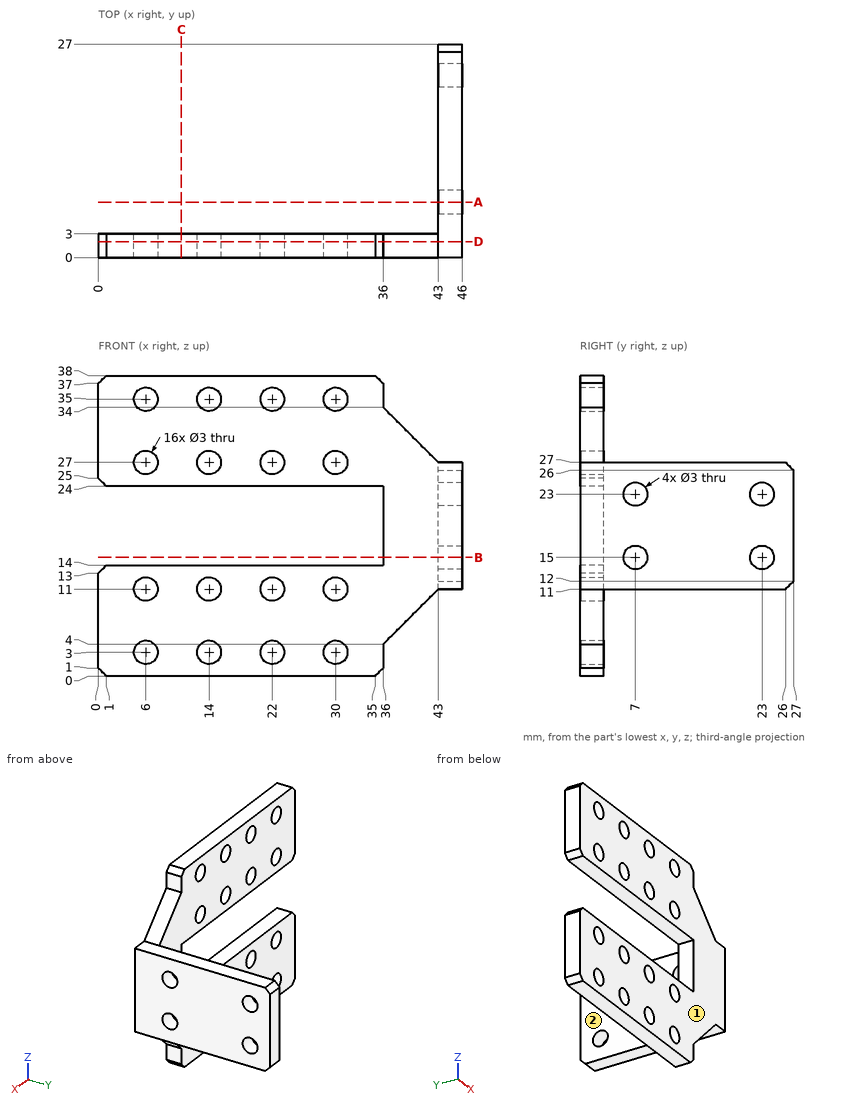
Could you check a few things on this drawing? It's one solid part, dimensions in mm from its lowest x, y, z. A direction names the side the tool comes from. Coordinates: 2 decimals unless noted, no trailing zeros. Loops run counter-clockwise (first coordinate to the right, second up) from the corner with the lowest first, then second, coordinate; pieces in that order, holes last. Notation, with made-up numbers: (77.5, -37) - (104.5, -37) arc R12 cw to (104.5, -30) - close; hole circle Ø11 at (44.25, -16.75). An arc over 180 degrees is marked (long way). Answer as a JSON object with one key per item and string values. Group by question number.
Item 1: If we section it at C-C (x = 10.5): List the corners of the cut face in (y, z) for me.
Item 2: If we section it at A-A (y = 7): List the corners of the cut face in (x, z) for me, plus the area to 3 significant figures.
Item 3: If we section it at D-D (y = 2): State how many separate pieces and enclosed holes the cut face has, plus the area to 3 significant figures.
Item 4: For pin 1 (2.5 mm diameter, centred on x = 30, z = 3, fed in from +Y); pin 2 (0.9 mm diameter, centred on y = 2, z = 16.5, fed in from -X); pin 3 (4 mm diameter, centred on x = 14, z = 11, fed in from +Y); pin 4 (4 mm diameter, centred on x = 22, z = 3, fed in from -Y), each with a flat end and sliding along its axis, tell me the tip position at first contact or that it passes through.
Item 5: On a 3-axis mill with a long thin cutter (end or side, diameter ignored), from which of +Z, -Z, +X, -X, +Y, -Y can I reach the whole of each face in a straight line? I mean the marked faces 1 and 2. Say none if no direction works.
Item 6: If I drill on L1, parallel to Z at x = 30, y = 1.35; L2, parallel to X at y = 0.6, z = 3; L3, parallel to Y at x = 10, z = 13, over which ranges is the centre line in solid material (lowest first)? Write a range as from..to.
Item 7: If we section it at B-B (z = 15): List the corners of the cut face in (x, y) for me, plus the area to 3 significant figures.
Returned:
{
 "1": {"outline": "(0, 0) - (3, 0) - (3, 14) - (0, 14) - close; (0, 24) - (3, 24) - (3, 38) - (0, 38) - close"},
 "2": {"outline": "(43, 11) - (46, 11) - (46, 13.5) - (43, 13.5) - close; (43, 16.5) - (46, 16.5) - (46, 21.5) - (43, 21.5) - close; (43, 24.5) - (46, 24.5) - (46, 27) - (43, 27) - close", "area": "30.0 mm²"},
 "3": {"separate pieces": "1", "enclosed holes": "16", "area": "1,100 mm²"},
 "4": {"pin 1": "passes through", "pin 2": "stops at x = 36", "pin 3": "stops at y = 3", "pin 4": "stops at y = 0"},
 "5": {"face 1": "+Z, -Z, +X, -X, -Y", "face 2": "+Z, -Z, -X, +Y"},
 "6": {"L1": "z = 0..1.5, 4.5..9.5, 12.5..14, 24..25.5, 28.5..33.5, 36.5..38", "L2": "x = 0..4.5, 7.5..12.5, 15.5..20.5, 23.5..28.5, 31.5..36", "L3": "y = 0..3"},
 "7": {"outline": "(36, 0) - (46, 0) - (46, 5.5) - (43, 5.5) - (43, 3) - (36, 3) - close; (43, 8.5) - (46, 8.5) - (46, 21.5) - (43, 21.5) - close; (43, 24.5) - (46, 24.5) - (46, 27) - (43, 27) - close", "area": "84.0 mm²"}
}
